from build123d import *

# Parameters (mm, degrees)
AUFSATZ_LINEAR_AUSTRAGEN1_DEPTH = 15
SKIZZE2_W                       = 50
SKIZZE2_H                       = 40
AUFSATZ_LINEAR_AUSTRAGEN2_DEPTH = 5
SKIZZE3_W                       = 11
SKIZZE3_H                       = 20
AUFSATZ_LINEAR_AUSTRAGEN3_DEPTH = 15


with BuildPart() as part:
    # Skizze1 → Aufsatz-Linear austragen1 (new body)
    with BuildSketch(Plane.XY):
        Polygon((8.642857143, 0), (-8.642857143, 0), (-12.5, -15), (-23.5, -15), (-5.5, 55), (5.5, 55), (23.5, -15), (12.5, -15), align=None)
        Polygon((0, 33.611111111), (-5.814285714, 11), (5.814285714, 11), align=None, mode=Mode.SUBTRACT)
    extrude(amount=AUFSATZ_LINEAR_AUSTRAGEN1_DEPTH)

    # Skizze2 → Aufsatz-Linear austragen2 (add)
    with BuildSketch(Plane.XZ.offset(15)):
        with Locations((0, 7.5)):
            Rectangle(SKIZZE2_W, SKIZZE2_H)
    extrude(amount=AUFSATZ_LINEAR_AUSTRAGEN2_DEPTH)

    # Skizze3 → Aufsatz-Linear austragen3 (add)
    with BuildSketch(Plane.XY.offset(15)):
        with Locations((0, 65)):
            Rectangle(SKIZZE3_W, SKIZZE3_H)
    extrude(amount=-AUFSATZ_LINEAR_AUSTRAGEN3_DEPTH)


solid = part.part
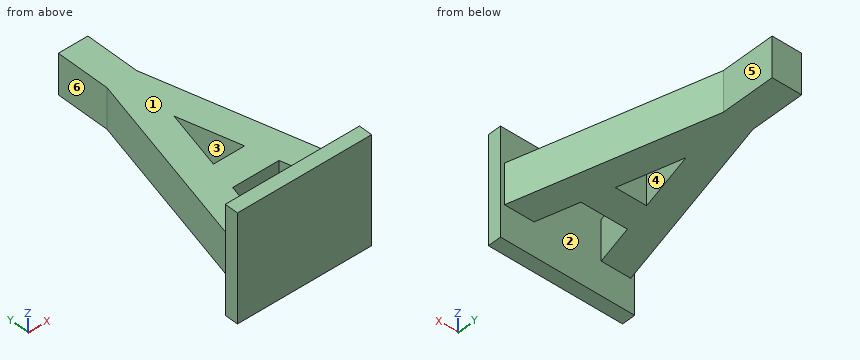
Geometry check sheet. Reference: the model listing, model coordinates, mm. Face numbers are marked on the shaded views. A direction names the side the tool comes from. Round coordinates to 2 decimals unless told otherwise and drop trailing zeros. Order: outer loops, then holes, each group sorted by start corner. A loop starts at its lowest first (then second) coordinate and runs counter-clockwise, first axis right, second up. Notation, with made-up numbers: M 18,62.5 L 76,62.5 A21 ccw 76,85.5 Z; hole C -33.75,29.25 d10. An arc over 180 degrees is marked long. Answer in a Markdown table with one row per item.
(1) Go/stop test with flat-tipped pins: P1, Ø6, axis at y = 60, z = 7.5, coming from the +X side; P2, Ø23.5, axis at x = -7.5, y = 46.5, coming from the -Z side; P3, Ø14, axis at x = -7.5, y = 29, coming from the +Z side; P4, Ø10, axis at y = 39, z = 21, coming from the -X side. Record where each tip stops, or that it passes through.
Responses:
| item | result |
|---|---|
| P1 | stops at x = 5.5 |
| P2 | stops at z = 0 |
| P3 | stops at z = 15 |
| P4 | passes through |
(2) Sectioned sample at C-C, the plane x = -19. Record the cut outline in (y, z).
Responses:
| item | result |
|---|---|
| outline | M -20,-12.5 L -15,-12.5 L -15,0 L 2.5,0 L 2.5,15 L -15,15 L -15,27.5 L -20,27.5 Z |
(3) Scan lines: probe 1 along Y at (x, z) = (9.5, -3.5); probe 2 along Z at (x, y) = (6.5, 15); probe 3 along X at (y, z) = (-2, 6). Record each from-to range of solid material in increasing order. Write a range as from..to.
Responses:
| item | result |
|---|---|
| probe 1 | y = -20..-15 |
| probe 2 | z = 0..15 |
| probe 3 | x = -20.16..-9.16, 9.16..20.16 |
(4) Draft check along X on the marked faces 4, 5 and 6. Enter one of: released by +X, released by -X, zero draft, split by the parting line, or undercut.
Responses:
| item | result |
|---|---|
| face 4 | undercut |
| face 5 | released by +X |
| face 6 | released by -X |
(5) Sectioned sample at A-A, the plane x = -3.5. Record the cut outline in (y, z).
Responses:
| item | result |
|---|---|
| outline | M -20,-12.5 L -15,-12.5 L -15,27.5 L -20,27.5 Z; M 0,0 L 11,0 L 11,15 L 0,15 Z; M 20,0 L 75,0 L 75,15 L 20,15 Z |
(6) Tool access check on the marked faces 1, 2 and 3. Record the directions out of +Z, -Z, +X, -X, +Y, -Y that give a thin tool (end or side, any length) a straight path to the whole face; none if there is none.
Responses:
| item | result |
|---|---|
| face 1 | +Z, +X, -X, +Y |
| face 2 | none |
| face 3 | +Z, -Z |
(7) Sectioned sample at B-B, the plane z = 1.5. Record the cut outline in (x, y).
Responses:
| item | result |
|---|---|
| outline | M -25,-20 L 25,-20 L 25,-15 L 23.5,-15 L 5.5,55 L 5.5,75 L -5.5,75 L -5.5,55 L -23.5,-15 L -25,-15 Z; hole M -12.5,-15 L 12.5,-15 L 8.64,0 L -8.64,0 Z; hole M -5.81,11 L 5.81,11 L 0,33.61 Z |
(8) Sectioned sample at D-D, the plane y = -6. Record the cut outline in (x, z), and give its area (3 significant figures).
Responses:
| item | result |
|---|---|
| outline | M -21.19,0 L -10.19,0 L -10.19,15 L -21.19,15 Z; M 10.19,0 L 21.19,0 L 21.19,15 L 10.19,15 Z |
| area | 330 mm² |
